Here's how the part is built. I have some questions about the finished solid (model axes, mm). Give positions to 0.01 mm unless a question says otherwise; leave off trailing zeros. Loops run counter-clockwise (first coordinate to the right, second up) from the corner with the lowest first, then second, coordinate; pieces in that order, holes last. Notation, with made-up numbers: (-28.5, 14.5) - (19.5, 14.5) arc R27 cw to (19.5, 37.5) - close; hole circle Ø11 at (-21, 11). An arc over 180 degrees is marked (long way). Put each result on its own line as item: value. Start each with the question number.
from build123d import *

# Parameters (mm, degrees)
F0_W           = 100
F0_H           = 80
F1_DEPTH       = 2.5
F2_R           = 25
F3_DEPTH       = 5
F4_R           = 30
F4_R_2         = 28
F5_DEPTH       = 1.5
F7_D           = 3.3
F7_CBORE_D     = 6.5
F7_CBORE_DEPTH = 3


with BuildPart() as f1:
    # F0 (on Top) → F1 (new body, symmetric)
    with BuildSketch(Plane.XY):
        Rectangle(F0_W, F0_H)
    extrude(amount=F1_DEPTH, both=True)

    # F2 (on face) → F3 (cut, through all)
    with BuildSketch(Plane.XY.offset(2.5)):
        Circle(F2_R)
    extrude(amount=-F3_DEPTH, mode=Mode.SUBTRACT)

    # F4 (on face) → F5 (cut)
    with BuildSketch(Plane.XY.offset(2.5)):
        Circle(F4_R)
        Circle(F4_R_2, mode=Mode.SUBTRACT)
    extrude(amount=-F5_DEPTH, mode=Mode.SUBTRACT)

    # F7 (through all)
    with Locations(Plane.XY.offset(2.5)):
        with Locations((-35, 35), (35, 35), (35, -35), (-35, -35)):
            CounterBoreHole(F7_D / 2, F7_CBORE_D / 2, F7_CBORE_DEPTH)


solid = f1.part
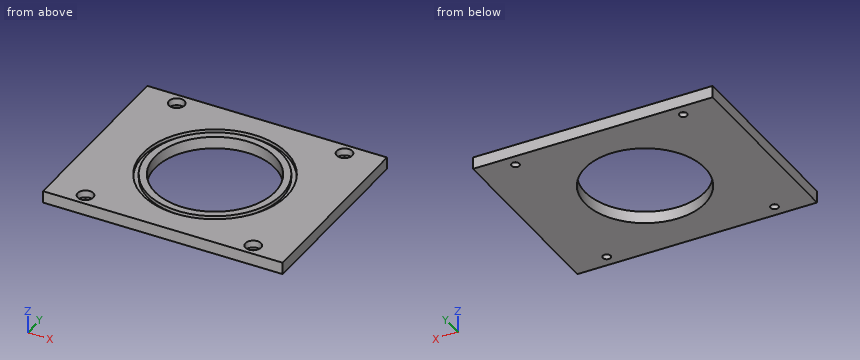
1) I'm going to push flat-ended pins straight in: P1, Ø2.5, axis at x = 35, y = -35, coming from the -Z side; P2, Ø2, axis at x = 36.5, y = 35, coming from the +Z side. Where does each tip first touch, or does it pass through?
2) Suppose I cut it at D-D on z = -1.5. Please give me the cut outline in (x, y), plus the area to 3 significant figures.
3) Suppose I cut it at A-A on x = 0. Please give me the cut outline in (y, z).
4) Suppose I cut it at B-B on x = -35. Please give me the cut outline in (y, z), plus the area to 3 significant figures.
5) I need wall thicknesses on line 1 (Y direction, x = 0, z = 2.15); line 2 (Y direction, x = 35, z = -1.35); line 3 (Y direction, x = -35, z = 1.2). Which ranges of each line are inside material? Lowest first, please.
6) Suppose I cut it at C-C on y = 35. Please give me the cut outline in (x, z), plus the area to 3 significant figures.
Ans:
1. P1: passes through
1. P2: stops at z = -0.5
2. outline: (-50, -40) - (50, -40) - (50, 40) - (-50, 40) - close; hole circle Ø3.3 at (-35, -35); hole circle Ø3.3 at (-35, 35); hole circle Ø50 at (0, 0); hole circle Ø3.3 at (35, -35); hole circle Ø3.3 at (35, 35)
2. area: 6,000 mm²
3. outline: (-40, -2.5) - (-25, -2.5) - (-25, 2.5) - (-28, 2.5) - (-28, 1) - (-30, 1) - (-30, 2.5) - (-40, 2.5) - close; (25, -2.5) - (40, -2.5) - (40, 2.5) - (30, 2.5) - (30, 1) - (28, 1) - (28, 2.5) - (25, 2.5) - close
4. outline: (-40, -2.5) - (-36.65, -2.5) - (-36.65, -0.5) - (-38.25, -0.5) - (-38.25, 2.5) - (-40, 2.5) - close; (-33.35, -2.5) - (33.35, -2.5) - (33.35, -0.5) - (31.75, -0.5) - (31.75, 2.5) - (-31.75, 2.5) - (-31.75, -0.5) - (-33.35, -0.5) - close; (36.65, -2.5) - (40, -2.5) - (40, 2.5) - (38.25, 2.5) - (38.25, -0.5) - (36.65, -0.5) - close
4. area: 348 mm²
5. line 1: y = -40 to -30, -28 to -25, 25 to 28, 30 to 40
5. line 2: y = -40 to -36.65, -33.35 to 33.35, 36.65 to 40
5. line 3: y = -40 to -38.25, -31.75 to 31.75, 38.25 to 40
6. outline: (-50, -2.5) - (-36.65, -2.5) - (-36.65, -0.5) - (-38.25, -0.5) - (-38.25, 2.5) - (-50, 2.5) - close; (-33.35, -2.5) - (33.35, -2.5) - (33.35, -0.5) - (31.75, -0.5) - (31.75, 2.5) - (-31.75, 2.5) - (-31.75, -0.5) - (-33.35, -0.5) - close; (36.65, -2.5) - (50, -2.5) - (50, 2.5) - (38.25, 2.5) - (38.25, -0.5) - (36.65, -0.5) - close
6. area: 448 mm²
